Input: part model. Units: mm. Frame: model coordinates. A direction names the side the tool comes from. Round coordinates to 2 decimals unless told otherwise and drop trailing zeros. Loops run counter-clockwise (first coordinate to the right, second up) from the corner with the lowest first, then second, coordinate; pieces in that order, holes last. Notation, with made-up numbers: M 11.5,88 L 27.5,88 A9 cw 27.5,92 Z; hole C -35.5,-4 d2. An arc over 180 degrees is marked long. Put each result on its own line as item: value. Start each with the question number.
1) Section A-A on x = -49.52. Output: boundary loops of the cut face in (y, z).
2) Section D-D on z = 8.5. State how many separate pieces and enclosed holes the cut face has, plus the area to 3 significant figures.
3) Reachability of faces 1 (the face through (8.767, -16.856, 4.93)), 2 (the face through (31, -8, 3)) from +Z, -Z, +X, -X, +Y, -Y: full face, straight path, thin tool, end or side. Return the list, or none.
4) Draft query along Y for faces 3 (the face through (30.41, -36.02, 4.93)), 4 (the face through (-14, 14, 10)). Return one class per face: +Y half, -Y half, draft (parallel to the pull), parting line (faces both ways), or undercut.
5) Section C-C on x = 33. Output: boundary loops of the cut face in (y, z).
6) Pin query (flat end, axial travel): pin 1 (6.5 mm diameter, centred on x = 33.59, y = 33.59, fed in from -Z); pin 2 (17.5 mm diameter, centred on x = 33, y = 0, fed in from +Z); pin 3 (5.5 mm diameter, centred on x = 24.74, y = 14.31, fed in from -Z); pin 4 (4 mm diameter, centred on y = 47.5, z = 7, fed in from +X). Return the tip coordinate at first contact, or that it passes through.
7) Line query: probe 1 along Y at (x, z) = (24, 7); probe 2 along Y at (x, z) = (45, 7.5); probe 3 along Y at (x, z) = (-30, 5). Output: solid intervals per line, ascending.
from build123d import *

# Parameters (mm, degrees)
SKETCH_R     = 60
SKETCH_R_2   = 2.1
SKETCH_R_3   = 19
SKETCH_R_4   = 8
SKETCH_R_5   = 4
PAD_DEPTH    = 10
SKETCH001_R  = 11
POCKET_DEPTH = 7
CHAMFER_SIZE = 2.2


with BuildPart() as part:
    # Sketch → Pad (new body)
    with BuildSketch(Plane.XY):
        Circle(SKETCH_R)
        with Locations((24.74, 14.30674)):
            Circle(SKETCH_R_2, mode=Mode.SUBTRACT)
        with Locations((24.74, -14.30674)):
            Circle(SKETCH_R_2, mode=Mode.SUBTRACT)
        Circle(SKETCH_R_3, mode=Mode.SUBTRACT)
        with Locations((33, 0)):
            Circle(SKETCH_R_4, mode=Mode.SUBTRACT)
        with Locations((49.52, 0)):
            Circle(SKETCH_R_2, mode=Mode.SUBTRACT)
        with Locations((-33.587572, 33.587572)):
            Circle(SKETCH_R_5, mode=Mode.SUBTRACT)
        with Locations((-33.587572, -33.587572)):
            Circle(SKETCH_R_5, mode=Mode.SUBTRACT)
        with Locations((33.587572, -33.587572)):
            Circle(SKETCH_R_5, mode=Mode.SUBTRACT)
        with Locations((33.587572, 33.587572)):
            Circle(SKETCH_R_5, mode=Mode.SUBTRACT)
        with Locations((-49.52, 0)):
            Circle(SKETCH_R_2, mode=Mode.SUBTRACT)
        with Locations((0, 49.52)):
            Circle(SKETCH_R_2, mode=Mode.SUBTRACT)
        with Locations((0, -49.52)):
            Circle(SKETCH_R_2, mode=Mode.SUBTRACT)
        with Locations((-43.487067, 23.688077)):
            Circle(SKETCH_R_2, mode=Mode.SUBTRACT)
        with Locations((-23.688077, 43.487067)):
            Circle(SKETCH_R_2, mode=Mode.SUBTRACT)
        with Locations((23.688077, -43.487067)):
            Circle(SKETCH_R_2, mode=Mode.SUBTRACT)
        with Locations((43.487067, -23.688077)):
            Circle(SKETCH_R_2, mode=Mode.SUBTRACT)
        with Locations((23.688077, 43.487067)):
            Circle(SKETCH_R_2, mode=Mode.SUBTRACT)
        with Locations((43.487067, 23.688077)):
            Circle(SKETCH_R_2, mode=Mode.SUBTRACT)
        with Locations((-43.487067, -23.688077)):
            Circle(SKETCH_R_2, mode=Mode.SUBTRACT)
        with Locations((-23.688077, -43.487067)):
            Circle(SKETCH_R_2, mode=Mode.SUBTRACT)
    extrude(amount=PAD_DEPTH)

    # Sketch001 (on Face23 of Pad) → Pocket (cut)
    with BuildSketch(Plane.XY.offset(10)):
        with Locations((33, 0)):
            Circle(SKETCH001_R)
    extrude(amount=-POCKET_DEPTH, mode=Mode.SUBTRACT)

    # Chamfer
    chamfer_edges = [part.edges().sort_by_distance(p)[0] for p in [
        (22.64, -14.30674, 0),
        (22.64, 14.30674, 0),
    ]]
    chamfer(chamfer_edges, length=CHAMFER_SIZE)


solid = part.part
Geometry results:
1. outline: M -33.88,0 L -2.1,0 L -2.1,10 L -33.88,10 Z; M 2.1,0 L 33.88,0 L 33.88,10 L 2.1,10 Z
2. separate pieces: 1
2. enclosed holes: 20
2. area: 9,400 mm²
3. face 1: +Z, -Z
3. face 2: +Z
4. face 3: undercut
4. face 4: draft
5. outline: M -50.11,0 L -37.54,0 L -37.54,10 L -50.11,10 Z; M -29.63,0 L -8,0 L -8,3 L -11,3 L -11,10 L -29.63,10 Z; M 8,0 L 29.63,0 L 29.63,10 L 11,10 L 11,3 L 8,3 Z; M 37.54,0 L 50.11,0 L 50.11,10 L 37.54,10 Z
6. pin 1: passes through
6. pin 2: stops at z = 3
6. pin 3: stops at z = 1.55
6. pin 4: stops at x = 39.11
7. probe 1: y = -54.99 to -45.56, -41.41 to -16.27, -12.34 to -6.32, 6.32 to 12.34, 16.27 to 41.41, 45.56 to 54.99
7. probe 2: y = -39.69 to -25.14, -22.23 to 22.23, 25.14 to 39.69
7. probe 3: y = -51.96 to -35.36, -31.82 to 31.82, 35.36 to 51.96
